```python
from build123d import *

# Parameters (mm, degrees)
SKETCH_R        = 10
PAD_DEPTH       = 30
SKETCH001_R     = 2.75
POCKET_DEPTH    = 30.001
SKETCH002_R     = 5
POCKET001_DEPTH = 10


with BuildPart() as part:
    # Sketch → Pad (new body)
    with BuildSketch(Plane.XY):
        Circle(SKETCH_R)
    extrude(amount=PAD_DEPTH)

    # Sketch001 (on Face3 of Pad) → Pocket (cut, through all)
    with BuildSketch(Plane.XY.offset(30)):
        Circle(SKETCH001_R)
    extrude(amount=-POCKET_DEPTH, mode=Mode.SUBTRACT)

    # Sketch002 (on Face3 of Pocket) → Pocket001 (cut)
    with BuildSketch(Plane.XY.offset(30)):
        Circle(SKETCH002_R)
    extrude(amount=-POCKET001_DEPTH, mode=Mode.SUBTRACT)


solid = part.part
```
Here's how the part is built. I have some questions about the finished solid (model axes, mm). A direction names the side the tool comes from. Round coordinates to 2 decimals unless told otherwise and drop trailing zeros. Loops run counter-clockwise (first coordinate to the right, second up) from the corner with the lowest first, then second, coordinate; pieces in that order, holes last. Notation, with made-up numbers: (40, 2) -> (72, 2) arc R16 cw to (72, 30) -> close; hole circle Ø8 at (89, -38). An arc over 180 degrees is marked (long way). Answer as CSV lines item,"result". Start each with the question number.
1. I'm going to push flat-ended pins straight in: P1, Ø4, axis at x = 7.5, z = 24, coming from the -Y side; P2, Ø5, axis at x = 0, y = 1.5, coming from the +Z side; P3, Ø1.5, axis at x = 7.5, z = 13.5, coming from the +Y side. Where does each tip first touch, or does it pass through?
2. Imagine slicing it at A-A on x = 0. Write out the boundary of the cut face in (y, z).
3. If we mould it in two halves opening along Y, with no side actions, what happens to faces 3 (the face through (-2.17, -9.76, 14.79)), 4 (the face through (-0.596, -2.685, 10.14)), 5 (the face through (2.1, -2.1, 0))? For each: pulls with the +Y half, pulls with the -Y half, needs draft (parallel to the pull), parting line crosses it, or undercut.
4. Imagine slicing it at C-C on z = 2.75. Write out the boundary of the cut face in (x, y).
5. I need wall thicknesses on probe 1 along Y at (x, z) = (0, 27); probe 2 along Y at (x, z) = (0, 11.75); probe 3 along X at (y, z) = (-1.5, 1.75). Which ranges of each line are inside material? Lowest first, please. Write a range as from..to.
6. For faces 1 (the face through (2.2, -2.2, 20)), 2 (the face through (-5, -2, 30)), which set-ups out of +Z, -Z, +X, -X, +Y, -Y let a thin tool reach every point of the face, with its end or its side?
7. Imagine slicing it at D-D on x = -4. Write out the boundary of the cut face in (y, z), plus the area to 3 significant figures.
Solution:
1,P1,"y = -8.35"
1,P2,"z = 20"
1,P3,"y = 7.38"
2,outline,"(-10, 0) -> (-2.75, 0) -> (-2.75, 20) -> (-5, 20) -> (-5, 30) -> (-10, 30) -> close; (2.75, 0) -> (10, 0) -> (10, 30) -> (5, 30) -> (5, 20) -> (2.75, 20) -> close"
3,face 3,"parting line crosses it"
3,face 4,"undercut"
3,face 5,"needs draft"
4,outline,"circle Ø20 at (0, 0); hole circle Ø5.5 at (0, 0)"
5,probe 1,"-10..-5, 5..10"
5,probe 2,"-10..-2.75, 2.75..10"
5,probe 3,"-9.89..-2.3, 2.3..9.89"
6,face 1,"+Z"
6,face 2,"+Z, +X, -X, +Y, -Y"
7,outline,"(-9.17, 0) -> (9.17, 0) -> (9.17, 30) -> (3, 30) -> (3, 20) -> (-3, 20) -> (-3, 30) -> (-9.17, 30) -> close"
7,area,"490 mm²"
